from build123d import *

# Parameters (mm, degrees)
F0_W     = 100
F0_H     = 50
F1_DEPTH = 35
F2_W     = 40
F2_H     = 60
F3_DEPTH = 95
F4_W     = 80
F4_H     = 10
F5_DEPTH = 5


with BuildPart() as f1:
    # F0 (on Top) → F1 (new body, symmetric)
    with BuildSketch(Plane.XY):
        with Locations((-50, 25)):
            Rectangle(F0_W, F0_H)
    extrude(amount=F1_DEPTH, both=True)

    # F2 (on face) → F3 (cut)
    with BuildSketch(Plane(origin=(-100, 0, 0), x_dir=(0, -1, 0), z_dir=(-1, 0, 0))):
        with Locations((-25, 0)):
            Rectangle(F2_W, F2_H)
    extrude(amount=-F3_DEPTH, mode=Mode.SUBTRACT)

    # F4 (on face) → F5 (cut, through all)
    with BuildSketch(Plane.XY.offset(35)):
        with Locations((-50, 25)):
            Rectangle(F4_W, F4_H)
    extrude(amount=-F5_DEPTH, mode=Mode.SUBTRACT)


solid = f1.part
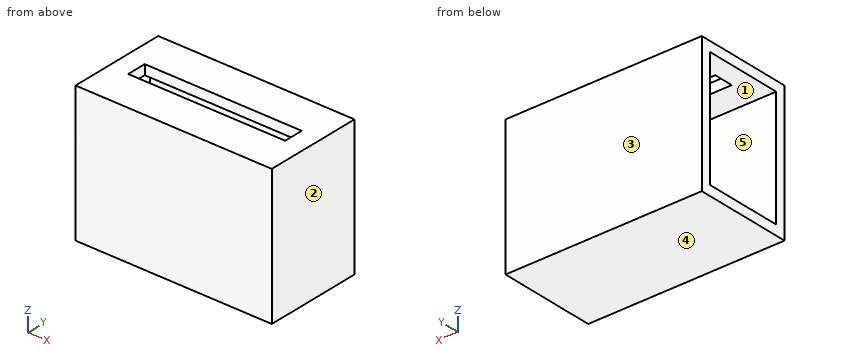
Could you check a few things on this model? Use its own coordinates, in mm. Face numbers are marked on the shaded views. A direction names the side the tool comes from. Coordinates: 2 decimals unless noted, no trailing zeros. Loops run counter-clockwise (first coordinate to the right, second up) from the corner with the lowest first, then second, coordinate; pieces in that order, holes last. Notation, with made-up numbers: (29.5, 83) -> (51.5, 83) arc R17 ccw to (51.5, 93) -> close; hole circle Ø8 at (25, 20). An arc over 180 degrees is marked (long way). Answer in a Markdown table with one row per item.
(1) Imagine slicing it at C-C (z = 25.5). List the corners of the cut face in (x, y) for me.
Results found:
| item | result |
|---|---|
| outline | (-100, 0) -> (0, 0) -> (0, 50) -> (-100, 50) -> (-100, 45) -> (-5, 45) -> (-5, 5) -> (-100, 5) -> close |
(2) Thinking about a two-plate mould opening in Y: for the marked faces 3, 4 and 5, which applies, released by +Y, released by -Y, zero draft, split by the parting line, or undercut?
Results found:
| item | result |
|---|---|
| face 3 | released by +Y |
| face 4 | zero draft |
| face 5 | undercut |
(3) Imagine slicing it at D-D (y = 36). List the corners of the cut face in (x, z) for me.
Results found:
| item | result |
|---|---|
| outline | (-100, -35) -> (0, -35) -> (0, 35) -> (-100, 35) -> (-100, 30) -> (-5, 30) -> (-5, -30) -> (-100, -30) -> close |
(4) Imagine slicing it at B-B (x = -92). List the corners of the cut face in (y, z) for me, plus the area to 3 significant figures.
Results found:
| item | result |
|---|---|
| outline | (0, -35) -> (50, -35) -> (50, 35) -> (0, 35) -> close; hole (5, -30) -> (45, -30) -> (45, 30) -> (5, 30) -> close |
| area | 1,100 mm^2 |
(5) Imagine slicing it at A-A (y = 24). List the corners of the cut face in (x, z) for me, plus the area to 3 significant figures.
Results found:
| item | result |
|---|---|
| outline | (-100, -35) -> (0, -35) -> (0, 35) -> (-10, 35) -> (-10, 30) -> (-5, 30) -> (-5, -30) -> (-100, -30) -> close; (-100, 30) -> (-90, 30) -> (-90, 35) -> (-100, 35) -> close |
| area | 900 mm^2 |
(6) Will these pins go through, and if not, where does the flat tip stop? pin 1 Ø5 at (y, z) = (12, -18.5) entering from -X; pin 2 Ø1.5 at (x, z) = (-69.5, 33.5) entering from -Y.
Results found:
| item | result |
|---|---|
| pin 1 | stops at x = -5 |
| pin 2 | stops at y = 0 |
(7) If I drill on probe 1 along Y at (x, z) = (-18, -0.5); probe 2 along X at (y, z) = (22.5, 30.5); probe 3 along Z at (x, y) = (-90, 36), over which ranges is the centre line in solid material (lowest first)?
Results found:
| item | result |
|---|---|
| probe 1 | y = 0 to 5, 45 to 50 |
| probe 2 | x = -100 to -90, -10 to 0 |
| probe 3 | z = -35 to -30, 30 to 35 |
(8) For the marked faces 1 and 2, which set-ups out of +Z, -Z, +X, -X, +Y, -Y let a thin tool reach every point of the face, with its end or its side?
Results found:
| item | result |
|---|---|
| face 1 | -X |
| face 2 | +Z, -Z, +X, +Y, -Y |
